The model under review builds one solid part; all positions refer to its coordinate system, in mm. A direction names the side the tool comes from. Coordinates: 2 decimals unless noted, no trailing zeros. Loops run counter-clockwise (first coordinate to the right, second up) from the corner with the lowest first, then second, coordinate; pieces in that order, holes last. Notation, with made-up numbers: (85.5, 67) -> (131.5, 67) arc R17 ccw to (131.5, 83) -> close; hole circle Ø7 at (37, 61.25). An arc over 180 degrees is marked (long way). One line per question, with ' | ' between items. Start each with the question number.
from build123d import *

# Parameters (mm, degrees)
F4_D     = 34.925
F6_D     = 6.985
F8_DEPTH = 66.04


with BuildPart() as f2:
    # F0 (on Right) → F2 (revolve)
    with BuildSketch(Plane.YZ):
        with BuildLine():
            Line((0, 23.8125), (0, 0))
            Line((0, 0), (66.04, 0))
            Line((66.04, 0), (66.04, 28.575))
            Line((66.04, 28.575), (34.29, 28.575))
            Line((34.29, 28.575), (34.29, 45.085))
            Line((34.29, 45.085), (27.94, 45.085))
            Line((27.94, 45.085), (27.94, 32.385))
            ThreePointArc((27.94, 32.385), (26.080128, 27.894872), (21.59, 26.035))
            Line((21.59, 26.035), (19.05, 26.035))
            Line((19.05, 26.035), (19.05, 23.8125))
            Line((19.05, 23.8125), (0, 23.8125))
        make_face()
    revolve(axis=Axis((0, 38.1, 0), (0, 1, 0)))

    # F4 (through all)
    with Locations(Plane.XZ):
        with Locations((0, 0)):
            Hole(F4_D / 2)

    # F6 (through all)
    with Locations(Plane.XZ.offset(-27.94)):
        with Locations((0, 36.5125), (31.620753, 18.25625), (31.620753, -18.25625), (0, -36.5125), (-31.620753, -18.25625), (-31.620753, 18.25625)):
            Hole(F6_D / 2)

    # F7 (on Front) → F8 (cut)
    with BuildSketch(Plane.XZ):
        Polygon((2.3495, 21.429623), (0, 21.429623), (-2.3495, 21.429623), (-2.3495, 16.803641), (0, 16.803641), (2.3495, 16.803641), align=None)
    extrude(amount=-F8_DEPTH, mode=Mode.SUBTRACT)


solid = f2.part
1) Mouldability with a two-part tool opening along X and no side actions: class faces 1 (the face through (0.45, 31.16, -33.05)), 2 (the face through (-14.49, 9.392, -18.897)), 3 (the face through (24, 27.94, 23)) as +X half, -X half, draft (parallel to the pull), parting line (faces both ways), or undercut.
2) Machinability: for faces 4 (the face through (-21.1, 19.05, 11.4)), 5 (the face through (-2.35, 33, 19)), 6 (the face through (-29, 34.29, 1)), 7 (the face through (13, 66.04, -12)), 8 (the face through (-14, 0, -11)), which of the approach directions +Z, -Z, +X, -X, +Y, -Y give a long, thin tool a straight path to every point of the face, cutting with its end or side? Answer none if there is none.
3) Wall thickness on L1, parallel to Z at x = -11, y = 25; L2, parallel to Z at x = -13.5, y = 3.5; L3, parallel to X at y = 24, z = -15.5: over which ranges is each line inside the solid? List them lowest first.
4) Consider section C-C, the plane x = 0. Give the number of separate pieces and of enclosed holes in the cut face, plus the area to 3 significant figures.
5) Insertion check: pin 1 Ø11 at (x, z) = (31.62, 18.26) entering from +Y; pin 2 Ø1.2 at (y, z) = (41, 19) entering from +X; pin 3 Ø6 at (y, z) = (29.5, 24) entering from -X; pin 4 Ø6.5 at (x, z) = (-31.62, 18.26) entering from +Y (3 decimals). Each pin has a flat end and moves straight along its axis. Give the tip position at first contact, or say it passes through.
6) Consider section D-D, the plane y = 16. Write out the cut boundary in (x, z) (1 decimal), plus the area to 3 significant figures.
Filled sheet:
1) face 1: undercut | face 2: parting line | face 3: draft
2) face 4: -Y | face 5: +Y, -Y | face 6: +Y | face 7: +Z, -Z, +X, -X, +Y | face 8: +Z, -Z, +X, -X, -Y
3) L1: -24.69 to -13.56, 13.56 to 24.69 | L2: -19.62 to -11.08, 11.08 to 19.62 | L3: -21.51 to -8.04, 8.04 to 21.51
4) separate pieces: 4 | enclosed holes: 0 | area: 1,120 mm^2
5) pin 1: y = 34.29 | pin 2: x = 21.86 | pin 3: x = -39.9 | pin 4: through
6) outline: circle Ø47.6 at (0, 0); hole (-2.3, 17.3) arc R17.5 ccw (long way) to (2.3, 17.3) -> (2.3, 21.4) -> (-2.3, 21.4) -> close | area: 805 mm^2
